Work out the finished part from the listing and answer in its coordinate system (mm). A direction names the side the tool comes from. Coordinates: 2 decimals unless noted, no trailing zeros. Write each loop counter-clockwise with the first axis right and the second up, starting at its lowest first coordinate (ties: lowest second). Pieces come first, ordered by that corner, then holes. Notation, with made-up numbers: M 82.5,3.25 L 101.5,3.25 A28 ccw 101.5,37.25 Z; hole C 61.5,22.25 d11. An arc over 180 degrees is marked long. Use CSV: the item, a comma, the result in double quotes.
from build123d import *

# Parameters (mm, degrees)
SKETCH1_W = 12
SKETCH1_H = 2


with BuildPart() as part:
    # Sketch1 → Revolve1 (revolve)
    with BuildSketch(Plane.XY, mode=Mode.PRIVATE) as revolve1_sk:
        Polygon((27.3, 2.5), (27.3, 2), (0, 2), (0, 0), (38.6, 0), (38.6, 2), (36.85, 2), (36.85, 1.9), (36.53, 1.9), (36.53, 2), (31.6, 2), (31.6, 2.5), align=None)
        with Locations((-6, 1)):
            Rectangle(SKETCH1_W, SKETCH1_H)
    revolve(revolve1_sk.sketch.rotate(Axis((0, 0, 0), (1, 0, 0)), 90), axis=Axis((0, 0, 0), (1, 0, 0)))


solid = part.part
Item 1: The part is cut by section A-A (z = 0). Write down the section's boundary in (x, y), then the cut area to 3 significant figures.
Answer:
outline,"M -12,-2 L 27.3,-2 L 27.3,-2.5 L 31.6,-2.5 L 31.6,-2 L 36.53,-2 L 36.53,-1.9 L 36.85,-1.9 L 36.85,-2 L 38.6,-2 L 38.6,2 L 36.85,2 L 36.85,1.9 L 36.53,1.9 L 36.53,2 L 31.6,2 L 31.6,2.5 L 27.3,2.5 L 27.3,2 L -12,2 Z"
area,"207 mm2"
Item 2: For a pull along X with two mould halves and no side action, classify faces 4 (the face through (38.6, 0, 0)), 5 (the face through (29.4, -0.1, -2.5)), 6 (the face through (36.688, -0.571, 1.812)) as released by +X, released by -X, zero draft, split by the parting line, or undercut.
Answer:
face 4,"released by +X"
face 5,"zero draft"
face 6,"undercut"
Item 3: A tool of negligible diameter and unlimited length cuts with its end or side. For faces 1 (the face through (34, 2, 0)), 2 (the face through (-12, 0, 0)), 3 (the face through (7, 2, 0)), from which of +Z, -Z, +X, -X, +Y, -Y can it reach the whole face along a straight path? Write none if from no direction.
Answer:
face 1,"+X"
face 2,"+Z, -Z, -X, +Y, -Y"
face 3,"-X"
Item 4: Consider probe 1 along X at (y, z) = (0.55, -2.3); probe 2 along Z at (x, y) = (20.5, -0.1); probe 3 along Y at (x, z) = (25.5, -0.2). Determine where each line is inside the solid, lowest interval first.
Answer:
probe 1,"x = 27.3 to 31.6"
probe 2,"z = -2 to 2"
probe 3,"y = -1.99 to 1.99"
Item 5: The part is cut by section C-C (x = 12). Write down the section's boundary in (y, z).
Answer:
outline,"C 0,0 d4"
Item 6: Given pin 1 (3 mm diameter, centred on x = 19.5, y = 0, fed in from -Z); pin 2 (3 mm diameter, centred on y = -1, z = -2, fed in from +X); pin 3 (3 mm diameter, centred on x = 15.5, y = 0, fed in from +Z); pin 4 (3 mm diameter, centred on x = -3.5, z = -0.5, fed in from -Y), each flat-ended and moving along its own axis, determine where each tip first touches the part or whether it passes through.
Answer:
pin 1,"stops at z = -2"
pin 2,"stops at x = 38.6"
pin 3,"stops at z = 2"
pin 4,"stops at y = -2"
